The listing builds one solid part. Answer for the finished solid, in the listing's coordinates (mm). Face numbers are marked on the shaded views. A direction names the side the tool comes from. Give positions to 0.01 mm unless a question says otherwise; leave off trailing zeros. Write each loop counter-clockwise with the first axis right and the second up, starting at its lowest first coordinate (ties: lowest second). Pieces come first, ordered by that corner, then holes. Notation, with made-up numbers: (68.5, 15) - (126.5, 15) arc R20 ccw to (126.5, 25) - close; hole circle Ø7 at (-5.75, -17). An arc over 180 degrees is marked (long way). Write each question's results on one line, items separated by ' | '. Start each with the question number.
Q1. Section A-A (y = 23) is taken. Determine the outline of the cut face in (x, z), plus the area to 3 significant figures.
Q2. For the marked faces 4, 5, 6, 7 and 8, determine the directions among +Z, -Z, +X, -X, +Y, -Y from which every point of the face is accessible in a straight line to the end or side of a thin tool.
Q3. Section D-D (x = -19.45) is taken. Determine the outline of the cut face in (y, z), plus the area to 3 significant figures.
Q4. Find the intervals of material crossed by probe 1 along Z at (x, y) = (-2.5, 14); probe 2 along Y at (x, z) = (-13.2, 0.75); probe 3 along Z at (x, y) = (-7, 5.75), in increasing order.
Q5. Flat-ended cylindrical pins translate along their axes: pin 1 Ø1.3 at (x, z) = (-20.5, 5) entering from -Y; pin 2 Ø1.3 at (y, z) = (18.5, 3.5) entering from +X; pin 3 Ø3 at (x, z) = (-3.5, -4) entering from -Y; pin 4 Ø1 at (y, z) = (6.5, 4) entering from -X. Find the tip coordinate at first contact, or state that the pin passes through.
Q6. For a pull along Y with two mould halves and no side action, classify the marked faces 1, 2 and 3 as pulls with the +Y half, pulls with the -Y half, needs draft (parallel to the pull), parting line crosses it, or undercut.
Q7. Section B-B (z = 4.05) is taken. Determine the outline of the cut face in (x, y).
Q8. Section C-C (x = -2.5) is taken. Determine the outline of the cut face in (y, z).
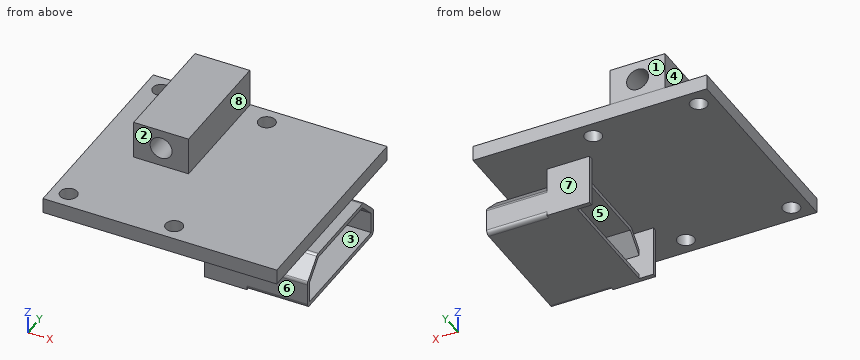
Autodesk Inventor part; units mm, degrees
ref_plane "YZ Plane" through (0, 0, 0) normal (1, 0, 0) x (0, 1, 0)
ref_plane "XZ Plane" through (0, 0, 0) normal (0, 1, 0) x (-1, 0, 0)
ref_plane "XY Plane" through (0, 0, 0) normal (0, 0, 1) x (1, 0, 0)
sketch "Sketch1" plane through (0, 0, 0) normal (0, 0, 1) x (1, 0, 0)
  line L0 (0, 0) -> (-27.7, 0)
  line L1 (-27.7, 0) -> (-27.7, 25)
  line L2 (-27.7, 25) -> (0, 25)
  line L3 (0, 25) -> (0, 0)
  circle A0 centre (-25.7, 23) radius 1
  circle A1 centre (-13.2, 23) radius 1
  circle A2 centre (-13.2, 2) radius 1
  circle A3 centre (-25.7, 2) radius 1
  line L4 (-25.7, 2) -> (-25.7, 23) construction
  line L5 (-25.7, 23) -> (-13.2, 23) construction
  line L6 (-13.2, 23) -> (-13.2, 2) construction
  line L7 (-13.2, 2) -> (-25.7, 2) construction
  line L8 (-13.2, 12.5) -> (0, 12.5) construction
  dimension "d0" = 25
  dimension "d1" = 27.7
  dimension "d2" = 12.5
  dimension "d3" = 21
  dimension "d4" = 2
  dimension "d5" = 2
extrude "Extrusion1" add sketch "Sketch1" along normal blind 1.8
sketch "Sketch2" plane through (0, 0, 1.8) normal (0, 0, 1) x (1, 0, 0)
  line L0 (0, 0) -> (0, 25) construction
  line L1 (0, 25) -> (-27.7, 25) construction
  line L2 (-27.7, 25) -> (-27.7, 0) construction
  line L3 (-27.7, 0) -> (0, 0) construction
  circle A0 centre (-25.7, 2) radius 1 construction
  circle A1 centre (-13.2, 2) radius 1 construction
  circle A2 centre (-13.2, 23) radius 1 construction
  circle A3 centre (-25.7, 23) radius 1 construction
  line L4 (-22.7, 11) -> (-16.2, 11)
  line L5 (-16.2, 11) -> (-16.2, 24.9)
  line L6 (-16.2, 24.9) -> (-22.7, 24.9)
  line L7 (-22.7, 24.9) -> (-22.7, 11)
  dimension "d8" = 6.5
  dimension "d10" = 5
  dimension "d33" = 14
  dimension "d34" = 0.1
extrude "Extrusion2" add sketch "Sketch2" along normal blind 4.5
ref_plane "Work Plane1" through (0, 25, 0) normal (0.7071, -0.7071, 0) x (0, 0, -1)
ref_plane "Work Plane2" through (-27.7, 26, 0) normal (0, 1, 0) x (1, 0, 0)
ref_plane "Work Plane3" through (1, 0, 0) normal (1, 0, 0) x (0, 0, -1)
sketch "Sketch4" plane through (1, 0, 0) normal (1, 0, 0) x (0, 0, -1)
  line L0 (5.5, 20) -> (3, 20)
  line L1 (0.5, 17.5) -> (0.5, 7.5)
  line L2 (3, 5) -> (5.5, 5)
  line L3 (6, 5.5) -> (6, 19.5)
  line L4 (0, 0) -> (0, 25) construction
  line L5 (2.6464, 19.8536) -> (0.6464, 17.8536)
  line L6 (2.6464, 5.1464) -> (0.6464, 7.1464)
  line L7 (6, 12.5) -> (0, 12.5) construction
  arc A0 (6, 19.5) -> (5.5, 20) centre (5.5, 19.5) ccw
  arc A1 (5.5, 5) -> (6, 5.5) centre (5.5, 5.5) ccw
  arc A2 (2.6464, 5.1464) -> (3, 5) centre (3, 5.5) ccw
  arc A3 (0.5, 7.5) -> (0.6464, 7.1464) centre (1, 7.5) ccw
  arc A4 (0.6464, 17.8536) -> (0.5, 17.5) centre (1, 17.5) ccw
  arc A5 (3, 20) -> (2.6464, 19.8536) centre (3, 19.5) ccw
  line L8 (5.5, 19.5) -> (5.5, 5.5)
  line L9 (5.5, 5.5) -> (3, 5.5)
  line L10 (3, 5.5) -> (1, 7.5)
  line L11 (1, 7.5) -> (1, 17.5)
  line L12 (1, 17.5) -> (3, 19.5)
  line L13 (3, 19.5) -> (5.5, 19.5)
  point P0 (6, 20)
  point P1 (6, 5)
  point P2 (0.5, 12.5)
  dimension "d17" = 0.5
  dimension "d19" = 15
  dimension "d20" = 5.5
  dimension "d21" = 0.5
  dimension "d22" = 135
  dimension "d23" = 3
  dimension "d24" = 0.5
extrude "Extrusion3" add sketch "Sketch4" against normal blind 10.5
sketch "Sketch5" plane through (1, 5.5, -6) normal (0, 0, -1) x (-1, 0, 0)
  line L0 (1, -5.5) -> (1, 19.5) construction
  line L1 (28.7, -5.5) -> (1, -5.5) construction
  line L2 (28.7, 19.5) -> (28.7, -5.5) construction
  line L3 (1, 19.5) -> (28.7, 19.5) construction
  circle A0 centre (26.7, -3.5) radius 1 construction
  circle A1 centre (14.2, -3.5) radius 1 construction
  circle A2 centre (14.2, 17.5) radius 1 construction
  circle A3 centre (26.7, 17.5) radius 1 construction
  line L4 (0, 0) -> (0, 14) construction
  line L5 (0, 0) -> (10.5, 0) construction
  line L6 (10.5, 14) -> (10.5, 0) construction
  line L7 (0, 14) -> (10.5, 14) construction
  line L8 (0, -0.5) -> (10.5, -0.5) construction
  line L9 (1, -5.5) -> (1, 19.5) construction
  line L10 (28.7, -5.5) -> (1, -5.5) construction
  line L11 (28.7, 19.5) -> (28.7, -5.5) construction
  line L12 (1, 19.5) -> (28.7, 19.5) construction
  circle A4 centre (26.7, -3.5) radius 1 construction
  circle A5 centre (14.2, -3.5) radius 1 construction
  circle A6 centre (14.2, 17.5) radius 1 construction
  circle A7 centre (26.7, 17.5) radius 1 construction
  line L13 (0, 14.5) -> (10.5, 14.5) construction
  line L14 (12.2, 14.5) -> (7.1495, 14.5)
  line L15 (7.1495, 14.5) -> (7.1495, 14)
  line L16 (7.1495, 14) -> (12.2, 14)
  line L17 (12.2, 14) -> (12.2, 14.5)
  line L18 (12.2, -0.5) -> (7.1495, -0.5)
  line L19 (7.1495, -0.5) -> (7.1495, 0)
  line L20 (7.1495, 0) -> (12.2, 0)
  line L21 (12.2, 0) -> (12.2, -0.5)
  dimension "d27" = 12.2
extrude "Extrusion4" add sketch "Sketch5" against normal up to surface (6 mm away)
sketch "Sketch6" plane through (-22.7, 11, 1.8) normal (0, -1, 0) x (1, 0, 0)
  line L0 (6.5, 0) -> (0, 0) construction
  line L1 (6.5, 0) -> (6.5, 4.5) construction
  line L2 (0, 4.5) -> (6.5, 4.5) construction
  line L3 (0, 0) -> (0, 4.5) construction
  line L4 (6.5, 0) -> (0, 4.5)
  circle A0 centre (3.25, 2.25) radius 1.3
  point P0 (22.7, -1.8)
  dimension "d30" = 2.6
extrude "Extrusion5" cut sketch "Sketch6" against normal through all
properties part number "F001-PCB1"
Answers below:
1) outline: (-27.7, 0) - (-26.7, 0) - (-26.7, 1.8) - (-27.7, 1.8) - close; (-24.7, 0) - (-14.2, 0) - (-14.2, 1.8) - (-16.2, 1.8) - (-16.2, 6.3) - (-22.7, 6.3) - (-22.7, 1.8) - (-24.7, 1.8) - close; (-12.2, 0) - (0, 0) - (0, 1.8) - (-12.2, 1.8) - close; hole circle Ø2.6 at (-19.45, 4.05) | area: 66.6 mm2
2) face 4: +Z, -X, +Y, -Y | face 5: +X, -X | face 6: -Z, +X, -X, -Y | face 7: -Z, +X, -X, +Y | face 8: +Z, +X, +Y, -Y
3) outline: (0, 0) - (25, 0) - (25, 1.8) - (24.9, 1.8) - (24.9, 2.75) - (11, 2.75) - (11, 1.8) - (0, 1.8) - close; (11, 5.35) - (24.9, 5.35) - (24.9, 6.3) - (11, 6.3) - close | area: 71.4 mm2
4) probe 1: z = -6 to -5.5, -1 to -0.5, 0 to 1.8 | probe 2: y = 0 to 1, 3 to 22, 24 to 25 | probe 3: z = -6 to -5.5, -2.75 to -2.04, 0 to 1.8
5) pin 1: stops at y = 11 | pin 2: stops at x = -16.2 | pin 3: stops at y = 5 | pin 4: passes through
6) face 1: pulls with the +Y half | face 2: pulls with the -Y half | face 3: undercut
7) outline: (-22.7, 11) - (-20.75, 11) - (-20.75, 24.9) - (-22.7, 24.9) - close; (-18.15, 11) - (-16.2, 11) - (-16.2, 24.9) - (-18.15, 24.9) - close
8) outline: (0, 0) - (25, 0) - (25, 1.8) - (0, 1.8) - close; (5, -5.5) arc R0.5 ccw to (5.5, -6) - (19.5, -6) arc R0.5 ccw to (20, -5.5) - (20, -3) arc R0.5 ccw to (19.85, -2.65) - (17.85, -0.65) arc R0.5 ccw to (17.5, -0.5) - (7.5, -0.5) arc R0.5 ccw to (7.15, -0.65) - (5.15, -2.65) arc R0.5 ccw to (5, -3) - close; hole (5.5, -5.5) - (19.5, -5.5) - (19.5, -3) - (17.5, -1) - (7.5, -1) - (5.5, -3) - close
